Input: dimensioned drawing with shaded views. Units: mm. Origin: part minimum x, y, z. Give positions to 0.01 mm unless a question says otherwise; leave off trailing zeros. Write each loop counter-clockwise with the first axis right and the second up, starting at its lowest first coordinate (ties: lowest second). Pieces come first, ordered by that corner, then holes. Notation, with made-up numbers: (88, 39) - (103, 39) arc R19 ccw to (103, 73) - close; hole circle Ø3 at (86.5, -35). An arc over 180 degrees is marked (long way). Answer as CSV lines item,"result".
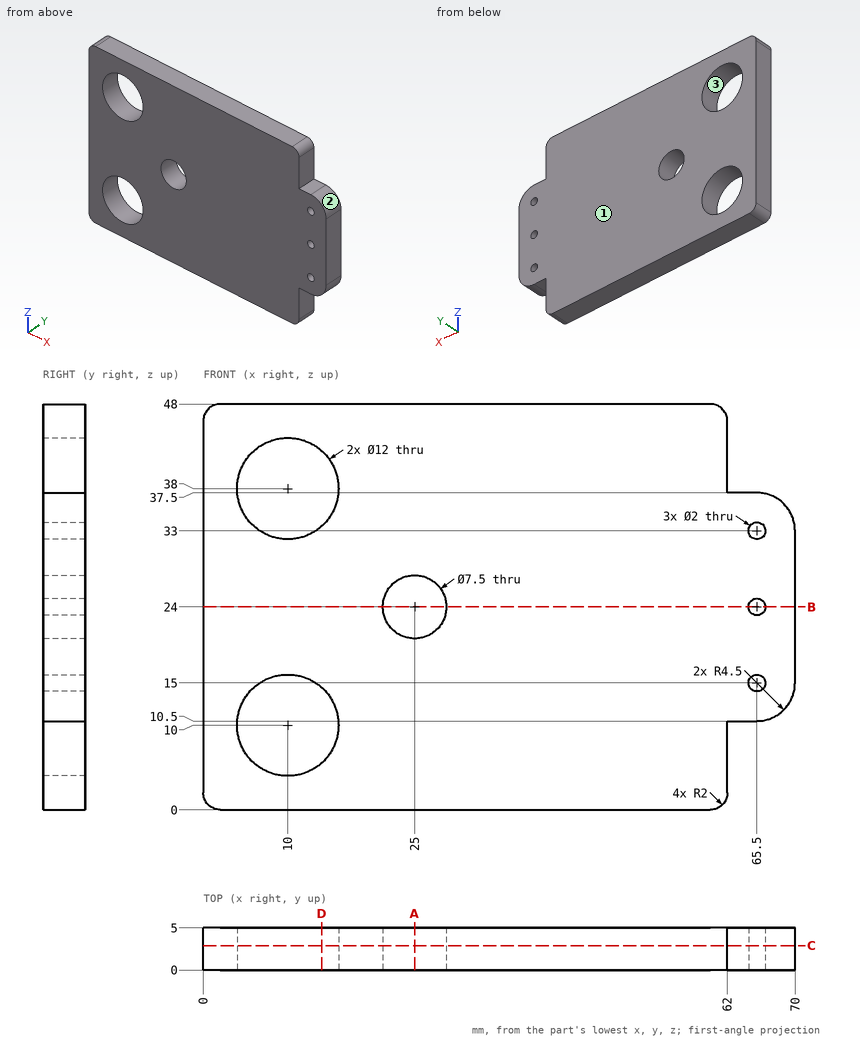
Item 1: Cut plane C-C on y = 2.9. Return the cut outline in (x, z).
The answers:
outline,"(0, 2) arc R2 ccw to (2, 0) - (60, 0) arc R2 ccw to (62, 2) - (62, 10.5) - (65.5, 10.5) arc R4.5 ccw to (70, 15) - (70, 33) arc R4.5 ccw to (65.5, 37.5) - (62, 37.5) - (62, 46) arc R2 ccw to (60, 48) - (2, 48) arc R2 ccw to (0, 46) - close; hole circle Ø12 at (10, 10); hole circle Ø12 at (10, 38); hole circle Ø7.5 at (25, 24); hole circle Ø2 at (65.5, 15); hole circle Ø2 at (65.5, 24); hole circle Ø2 at (65.5, 33)"
Item 2: Contact query for flat-ended pins moving along their axis: pin 1 (14 mm diameter, centred on x = 10, z = 10, fed in from -Y); pin 2 (1.8 mm diameter, centred on x = 65.5, z = 15, fed in from -Y); pin 3 (1.8 mm diameter, centred on x = 64.5, y = 1.5, fed in from +Z); pin 4 (1.8 mm diameter, centred on x = 63.5, y = 1.5, fed in from -Z). Output: stop coordinate, or through.
The answers:
pin 1,"y = 0"
pin 2,"through"
pin 3,"z = 37.5"
pin 4,"z = 10.5"
Item 3: Ray query, line 1 (X direction, y = 2.6, z = 24); line 2 (Z direction, x = 5, y = 3.2); line 3 (Z direction, x = 9, y = 1.1). Return the intervals inside material, ascending. Write a range as from..to.
The answers:
line 1,"0..21.25, 28.75..64.5, 66.5..70"
line 2,"0..6.68, 13.32..34.68, 41.32..48"
line 3,"0..4.08, 15.92..32.08, 43.92..48"
Item 4: Cut plane A-A on x = 25. Return the cut outline in (y, z), plus the area to 4 significant figures.
The answers:
outline,"(0, 0) - (5, 0) - (5, 20.25) - (0, 20.25) - close; (0, 27.75) - (5, 27.75) - (5, 48) - (0, 48) - close"
area,"202.5 mm²"
Item 5: Cut plane B-B on z = 24. Return the cut outline in (x, y).
The answers:
outline,"(0, 0) - (21.25, 0) - (21.25, 5) - (0, 5) - close; (28.75, 0) - (64.5, 0) - (64.5, 5) - (28.75, 5) - close; (66.5, 0) - (70, 0) - (70, 5) - (66.5, 5) - close"
Item 6: Cut plane D-D on x = 14. Return the cut outline in (y, z), plus the area to 3 significant figures.
The answers:
outline,"(0, 0) - (5, 0) - (5, 5.53) - (0, 5.53) - close; (0, 14.47) - (5, 14.47) - (5, 33.53) - (0, 33.53) - close; (0, 42.47) - (5, 42.47) - (5, 48) - (0, 48) - close"
area,"151 mm²"
Item 7: Mould query, pull axis X, two halves, no side actions, for the marked faces 1, 2 and 3. Classes: +X half, -X half, draft (parallel to the pull), parting line (faces both ways), or undercut.
The answers:
face 1,"draft"
face 2,"+X half"
face 3,"undercut"
